```python
from build123d import *

# Parameters (mm, degrees)
SZKIC2_R                    = 2.5
DODANIE_WYCI_GNI_CIE3_DEPTH = 2


with BuildPart() as part:
    # Szkic2 → Dodanie-wyci_gni_cie3 (new body)
    with BuildSketch(Plane.XY):
        with BuildLine():
            Line((-32, -20), (32, -20))
            ThreePointArc((32, -20), (34.121320344, -19.121320344), (35, -17))
            Line((35, -17), (35, 17))
            ThreePointArc((35, 17), (34.121320344, 19.121320344), (32, 20))
            Line((32, 20), (-32, 20))
            ThreePointArc((-32, 20), (-34.121320344, 19.121320344), (-35, 17))
            Line((-35, 17), (-35, -17))
            ThreePointArc((-35, -17), (-34.121320344, -19.121320344), (-32, -20))
        make_face()
        with Locations((-27, 14.666666667)):
            Circle(SZKIC2_R, mode=Mode.SUBTRACT)
        with Locations((27.540515543, -1.488970059)):
            Circle(SZKIC2_R, mode=Mode.SUBTRACT)
        with Locations((-24.693752651, -14.408678002)):
            Circle(SZKIC2_R, mode=Mode.SUBTRACT)
        with BuildLine():
            ThreePointArc((7.175560187, -9.273316659), (9.665957804, -5.250643745), (11.684967283, -0.97190814))
            ThreePointArc((11.684967283, -0.97190814), (5.609428267, 13.3489796), (-8.711459473, 7.273440584))
            ThreePointArc((-8.711459473, 7.273440584), (-9.665957804, 5.250643745), (-10.843307584, 3.348902015))
            ThreePointArc((-10.843307584, 3.348902015), (-8.144983036, -11.971641207), (7.175560187, -9.273316659))
        make_face(mode=Mode.SUBTRACT)
    extrude(amount=DODANIE_WYCI_GNI_CIE3_DEPTH)


solid = part.part
```
Check sheet for the modelled part. Datum: model origin and axes. Units: mm. A direction names the side the tool comes from. Coordinates: 2 decimals unless noted, no trailing zeros. Order: outer loops, then holes, each group sorted by start corner. A loop starts at its lowest first (then second) coordinate and runs counter-clockwise, first axis right, second up. Notation, with made-up numbers: M -31,4.25 L -11,4.25 A19 cw -11,11.25 Z; hole C 85,3 d1. An arc over 180 degrees is marked long. Write each question's results on one line, items separated by ' | '. Start each with the question number.
1. Cross-section at B-B on z = 0.9. Record the cut outline in (x, y), and give its area (3 significant figures).
2. Access from +Z, -Z, +X, -X, +Y, -Y to the whole of each face (thin tool, end or side, straight path). Record for faces 1 (the face through (9.634, -5.309, 0.986)), 2 (the face through (34.1, -19.14, 0.99)).
3. Material ranges on probe 1 along Y at (x, z) = (-27, 0.65); probe 2 along Y at (x, z) = (-8, 0.3); probe 3 along Y at (x, z) = (-23.5, 0.7), recorded low to high.
4. Cross-section at C-C on y = 13. Record the cut outline in (x, z), and give its area (3 significant figures).
5. Cross-section at D-D on x = 8.5. Record the cut outline in (y, z), and give its area (3 significant figures).
6. Cross-section at A-A on x = 27. Record the cut outline in (y, z).
7. Mould release check, pull along X, two halves, no side actions. Record for faces 3 (the face through (0, 20, 1)), 4 (the face through (34.14, 19.1, 0.99)), 5 (the face through (25.557, -3.01, 0.986)): +X half, -X half, draft (parallel to the pull), parting line (faces both ways), or undercut.
8. Go/stop test with flat-tipped pins: P1, Ø8, axis at x = 26, y = 16, coming from the -Z side; P2, Ø4.5, axis at x = -24.69, y = -14.41, coming from the -Z side. Record where each tip stops, or that it passes through.
Checks:
1) outline: M -35,-17 A3 ccw -32,-20 L 32,-20 A3 ccw 35,-17 L 35,17 A3 ccw 32,20 L -32,20 A3 ccw -35,17 Z; hole C -27,14.67 d5; hole C -24.69,-14.41 d5; hole M -10.84,3.35 A11 ccw 7.18,-9.27 A41.73 ccw 11.68,-0.97 A11 ccw -8.71,7.27 A19.73 cw Z; hole C 27.54,-1.49 d5 | area: 2,200 mm²
2) face 1: +Z, -Z | face 2: +Z, -Z, +X, -Y
3) probe 1: y = -20 to -15.37, -13.44 to 12.17, 17.17 to 20 | probe 2: y = -20 to -12.07, 8.72 to 20 | probe 3: y = -20 to -16.61, -12.21 to 20
4) outline: M -35,0 L -28.86,0 L -28.86,2 L -35,2 Z; M -25.14,0 L -3.41,0 L -3.41,2 L -25.14,2 Z; M 6.38,0 L 35,0 L 35,2 L 6.38,2 Z | area: 113 mm²
5) outline: M -20,0 L -7.26,0 L -7.26,2 L -20,2 Z; M 11.63,0 L 20,0 L 20,2 L 11.63,2 Z | area: 42.2 mm²
6) outline: M -20,0 L -3.93,0 L -3.93,2 L -20,2 Z; M 0.95,0 L 20,0 L 20,2 L 0.95,2 Z
7) face 3: draft | face 4: +X half | face 5: undercut
8) P1: stops at z = 0 | P2: passes through
